Autodesk Inventor part; units mm, degrees
ref_plane "YZ Plane" through (0, 0, 0) normal (1, 0, 0) x (0, 1, 0)
ref_plane "XZ Plane" through (0, 0, 0) normal (0, 1, 0) x (-1, 0, 0)
ref_plane "XY Plane" through (0, 0, 0) normal (0, 0, 1) x (1, 0, 0)
sketch "Sketch1" plane through (0, 0, 0) normal (0, 1, 0) x (-1, 0, 0)
  line L0 (0, 0) -> (-101.6, 0)
  line L1 (-101.6, 0) -> (-101.6, 304.8)
  line L2 (-101.6, 304.8) -> (0, 304.8)
  line L3 (0, 304.8) -> (0, 0)
  point P0 (-50.8, 152.4)
  dimension "d0" = 101.6
  dimension "d1" = 304.8
  dimension "d25" = 50.8
  dimension "d26" = 152.4
extrude "Extrusion1" add sketch "Sketch1" along normal blind 6.35
hole "Hole2" at (26.9875, 6.35, 152.4) direction (0, -1, 0) diameter 4.8768 end through all
hole "Hole3" at (50.8, 6.35, 152.4) direction (0, -1, 0) diameter 6.35 end through all
pattern_circular "Circular Pattern2" count 6 over 360 about axis through (50.8, -315.0002, 152.4) along (0, 1, 0) of "Hole2"
properties part number "Claw Plate"
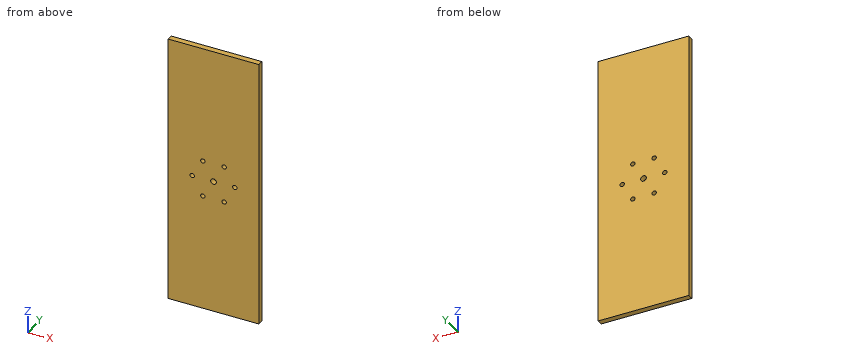
The model under review builds one solid part; all positions refer to its coordinate system, in mm. Round coordinates to 2 decimals unless told otherwise and drop trailing zeros. Order: outer loops, then holes, each group sorted by start corner. A loop starts at its lowest first (then second) coordinate and runs counter-clockwise, first axis right, second up. Notation, with made-up numbers: (41.5, 37.5) -> (97.5, 37.5) arc R29 cw to (97.5, 68.5) -> close; hole circle Ø2 at (42.5, -33.75). An arc over 180 degrees is marked (long way). One line per item, written item: value. Start each with the question number.
Q1. Take a section at A-A (x = 50.8). Write out the cut boundary in (y, z) (3 decimals).
Q2. Clearance check with a flat-ended pin moving along its axis: pin 1 Ø4.5 at (x, z) = (38.89, 173.02) entering from +Y. State where the tip first meets the part, or that it passes through.
Q3. Wall thickness on line 1 (Z direction, x = 63, y = 1.75); line 2 (X direction, y = 2.5, z = 152.4) (3 decimals); line 3 (Z direction, x = 38, y = 1.5): over which ranges is each line inside the solid? List them lowest first.
Reported:
1. outline: (0, 0) -> (6.35, 0) -> (6.35, 149.225) -> (0, 149.225) -> close; (0, 155.575) -> (6.35, 155.575) -> (6.35, 304.8) -> (0, 304.8) -> close
2. pin 1: passes through
3. line 1: z = 0 to 129.36, 134.2 to 170.6, 175.44 to 304.8
3. line 2: x = 0 to 24.549, 29.426 to 47.625, 53.975 to 72.174, 77.051 to 101.6
3. line 3: z = 0 to 129.51, 134.05 to 170.75, 175.29 to 304.8
